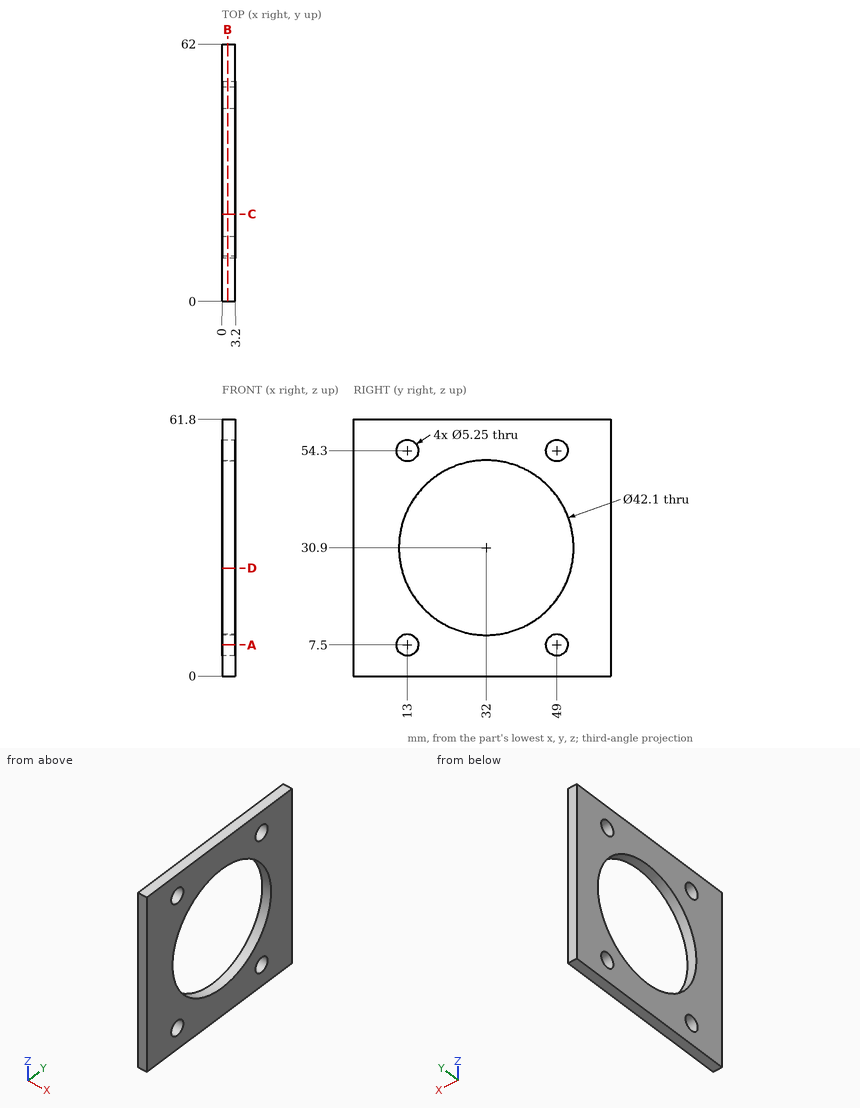
Input: dimensioned drawing with shaded views. Units: mm. Origin: part minimum x, y, z. Coordinates: 2 decimals unless noted, no trailing zeros. Write each loop counter-clockwise with the first axis right and the second up, starting at its lowest first coordinate (ties: lowest second). Pieces come first, ordered by that corner, then holes. Notation, with made-up numbers: (-7.5, -36) -> (3.5, -36) arc R15 ccw to (3.5, -13) -> close; hole circle Ø1 at (27, 42.5). An arc over 180 degrees is marked (long way). Return JSON: item names as keys, results as strings. Group by question number.
1) Section query B-B, the plane x = 1.3. Return loops of the section in (y, z) (3 decimals).
2) Section query C-C, the plane y = 21. Return loops of the section in (x, z).
3) Section query A-A, the plane z = 7.5. Return loops of the section in (x, y) (3 decimals), plus the area to 3 significant figures.
4) Ray query, line 1 along Y through (x, z) = (1.85, 54.3) (3 decimals); line 2 along Z through (x, y) = (0.6, 50); line 3 along Y through (x, z) = (2.1, 30.9). Return the intervals inside material, ascending.
5) Contact query for a flat-ended pin moving along its axis: P1, Ø4, axis at y = 13, z = 54.3, coming from the +X side. Output: stop coordinate, or through.
6) Section query D-D, the plane z = 26. Return loops of the section in (x, y).
From the geometry:
{
 "1": {"outline": "(0, 0) -> (62, 0) -> (62, 61.8) -> (0, 61.8) -> close; hole circle Ø5.25 at (13, 7.5); hole circle Ø5.25 at (13, 54.3); hole circle Ø42.1 at (32, 30.9); hole circle Ø5.25 at (49, 7.5); hole circle Ø5.25 at (49, 54.3)"},
 "2": {"outline": "(0, 0) -> (3.2, 0) -> (3.2, 12.95) -> (0, 12.95) -> close; (0, 48.85) -> (3.2, 48.85) -> (3.2, 61.8) -> (0, 61.8) -> close"},
 "3": {"outline": "(0, 0) -> (3.2, 0) -> (3.2, 10.375) -> (0, 10.375) -> close; (0, 15.625) -> (3.2, 15.625) -> (3.2, 46.375) -> (0, 46.375) -> close; (0, 51.625) -> (3.2, 51.625) -> (3.2, 62) -> (0, 62) -> close", "area": "165 mm²"},
 "4": {"line 1": "0 to 10.375, 15.625 to 46.375, 51.625 to 62", "line 2": "0 to 5.07, 9.93 to 19.99, 41.81 to 51.87, 56.73 to 61.8", "line 3": "0 to 10.95, 53.05 to 62"},
 "5": {"P1": "through"},
 "6": {"outline": "(0, 0) -> (3.2, 0) -> (3.2, 11.53) -> (0, 11.53) -> close; (0, 52.47) -> (3.2, 52.47) -> (3.2, 62) -> (0, 62) -> close"}
}
